```python
from build123d import *

# Parameters (mm, degrees)
BOSS_EXTRUDE2_DEPTH     = 222.25
SKETCH4_W               = 3.175
SKETCH4_H               = 9.525
SKETCH4_W_2             = 11.35728502
SKETCH4_H_2             = 30.48
CUT_EXTRUDE2_DEPTH      = 20.034637206
CUT_EXTRUDE2_DEPTH_BACK = 28.684375793


with BuildPart() as part:
    # Sketch3 → Boss-Extrude2 (new body)
    with BuildSketch(Plane(origin=(0, 0, 0), x_dir=(1, 0, 0), z_dir=(0, 1, 0))):
        Polygon((-37.062566366, 21.904788086), (-19.755538483, 15.964920897), (0, 0), (12.541749156, -4.304397313), (21.323689681, -5.686287551), (21.57426256, -4.093891817), (12.792322036, -2.712001578), (0.780092903, 1.410661549), (-18.975445581, 17.375582446), (-37.062566366, 23.583181811), align=None)
    extrude(amount=BOSS_EXTRUDE2_DEPTH)

    # Sketch4 → Cut-Extrude2 (cut, two sides)
    with BuildSketch(Plane(origin=(3.335400558, 0, -9.718377301), x_dir=(-0.945844814, 0, -0.324619144), z_dir=(0.324619144, 0, -0.945844814))) as cut_extrude2_sk:
        with Locations((41.123488466, 131.1275)):
            Rectangle(SKETCH4_W, SKETCH4_H)
        Polygon((42.710988466, 95.885), (42.710988466, 126.365), (39.535988466, 126.365), (23.588273486, 126.365), (23.588273486, 95.885), (39.535988466, 95.885), align=None)
        with Locations((41.123488466, 91.1225)):
            Rectangle(SKETCH4_W, SKETCH4_H)
        with Locations((17.909630976, 111.125)):
            Rectangle(SKETCH4_W_2, SKETCH4_H_2)
    extrude(amount=CUT_EXTRUDE2_DEPTH, mode=Mode.SUBTRACT)
    extrude(cut_extrude2_sk.sketch, amount=-CUT_EXTRUDE2_DEPTH_BACK, mode=Mode.SUBTRACT)


solid = part.part
```
Verification items for the finished model (mm, model axes). Round coordinates to 2 decimals unless told otherwise and drop trailing zeros. Write each loop counter-clockwise with the first axis right and the second up, starting at its lowest first coordinate (ties: lowest second). Pieces come first, ordered by that corner, then holes.
1. Section check C-C on y = 130.5. Enter the section's corners in (x, z), plus the area to 3 significant figures.
2. Section check A-A on z = -11.75. Enter the section's corners in (x, y) (3 decimals).
3. Section check B-B on x = -14. Enter the section's corners in (y, z) (3 decimals), plus the area to 3 significant figures.
4. Gauge pin test, flat ends, axial feed: P1, Ø12, axis at y = 46.5, z = -14, coming from the +X side; P2, Ø6, axis at x = -12.5, y = 194.5, coming from the -Z side; P3, Ø8, axis at x = 13, y = 55, coming from the -Z side. Record the tip position at first contact, or that the pin passes through.
5. Section check D-D on y = 176. Enter the section's corners in (x, z), plus the area to 3 significant figures.
6. Draft check along Y on faces 1 (the flat face through (16.871, 109.569, 4.986)), 2 (the flat face through (-8, 0, -8)), 3 (the flat face through (-21, 95.885, -17)). Enter one of: +Y half, -Y half, draft (parallel to the pull), parting line (faces both ways), or undercut.
7. Scan lines: L1, parallel to Z at x = -24, y = 95.5; L2, parallel to X at y = 92.5, z = -10.75; L3, parallel to X at y = 177.5, z = -15.5. Record each from-to range of solid material in increasing order.
Answer:
1. outline: (-34.57, -21.05) - (-34.06, -22.55) - (-18.98, -17.38) - (0.78, -1.41) - (12.79, 2.71) - (21.57, 4.09) - (21.32, 5.69) - (12.54, 4.3) - (0, 0) - (-19.76, -15.96) - close
1. area: 100 mm2
2. outline: (-14.54, 0) - (-12.014, 0) - (-12.014, 95.885) - (-14.54, 95.885) - close; (-14.54, 126.365) - (-12.014, 126.365) - (-12.014, 222.25) - (-14.54, 222.25) - close
3. outline: (0, -13.355) - (95.885, -13.355) - (95.885, -11.314) - (0, -11.314) - close; (126.365, -13.355) - (222.25, -13.355) - (222.25, -11.314) - (126.365, -11.314) - close
3. area: 391 mm2
4. P1: stops at x = -7.37
4. P2: stops at z = -14.57
4. P3: stops at z = 1.41
5. outline: (-37.06, -23.58) - (-18.98, -17.38) - (0.78, -1.41) - (12.79, 2.71) - (21.57, 4.09) - (21.32, 5.69) - (12.54, 4.3) - (0, 0) - (-19.76, -15.96) - (-37.06, -21.9) - close
5. area: 105 mm2
6. face 1: draft
6. face 2: -Y half
6. face 3: undercut
7. L1: z = -19.1 to -17.42
7. L2: x = -13.3 to -10.78
7. L3: x = -19.18 to -16.65
